```python
from build123d import *

# Parameters (mm, degrees)
SKETCH1_W           = 15.25
SKETCH1_H           = 10
SKETCH1_R           = 1.15
SKETCH1_R_2         = 0.381
BOSS_EXTRUDE1_DEPTH = 1.5
FILLET2_R           = 2


with BuildPart() as part:
    # Sketch1 → Boss-Extrude1 (new body)
    with BuildSketch(Plane(origin=(0, 0, 0), x_dir=(1, 0, 0), z_dir=(0, 1, 0))):
        with Locations((7.625, 5)):
            Rectangle(SKETCH1_W, SKETCH1_H)
        with Locations(Location((12.755741127, 5, 0), (0, 0, 270))):
            Circle(SKETCH1_R, mode=Mode.SUBTRACT)
        with Locations(Location((2, 6.27, 0), (0, 0, 270))):
            Circle(SKETCH1_R_2, mode=Mode.SUBTRACT)
        with Locations(Location((2, 3.73, 0), (0, 0, 270))):
            Circle(SKETCH1_R_2, mode=Mode.SUBTRACT)
        with Locations(Location((2, 1.19, 0), (0, 0, 270))):
            Circle(SKETCH1_R_2, mode=Mode.SUBTRACT)
        with Locations(Location((2, 8.81, 0), (0, 0, 270))):
            Circle(SKETCH1_R_2, mode=Mode.SUBTRACT)
    extrude(amount=BOSS_EXTRUDE1_DEPTH)

    # Fillet2
    fillet2_edges = [part.edges().sort_by_distance(p)[0] for p in [
        (15.25, 0.75, -10),
        (15.25, 0.75, 0),
    ]]
    fillet(fillet2_edges, radius=FILLET2_R)


solid = part.part
```
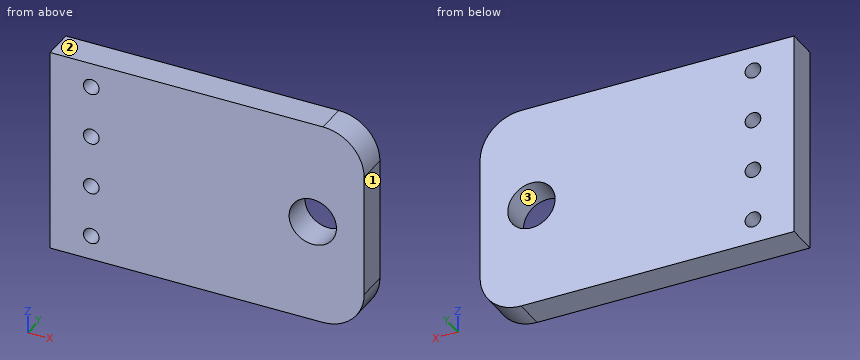
The listing builds one solid part. Answer for the finished solid, in the listing's coordinates (mm). Face numbers are marked on the shaded views. Round coordinates to 2 decimals unless told otherwise and drop trailing zeros. Order: outer loops, then holes, each group sorted by start corner. A loop starts at its lowest first (then second) coordinate and runs counter-clockwise, first axis right, second up. Notation, with made-up numbers: (28, 9) - (65, 9) arc R25 cw to (65, 34) - close; hole circle Ø11 at (80, -7). An arc over 180 degrees is marked (long way). Put each result on its own line as item: value. Start each with the question number.
(1) Determine the mould class of the marked faces 1, 2 and 3 for opening direction X: released by +X, released by -X, zero draft, split by the parting line, or undercut.
(2) Straight lines are drawn through the part: probe 1 along X at (y, z) = (1.45, -6.25); probe 2 along X at (y, z) = (0.3, -4); probe 3 along X at (y, z) = (0.95, -8.81). For each, find the intervals that lie inside material, in ascending order. Write a range as from..to.
(3) Find section B-B (z = -8.81). Give the vertices of the cut face in (x, y), plus the area to 3 significant figures.
(4) Find section A-A (x = 2). Give the vertices of the cut face in (y, z).
(5) Find section C-C (y = 0.9). Give the vertices of the cut face in (x, z), plus the area to 3 significant figures.
(6) Find section D-D (x = 14.25). Give the vertices of the cut face in (y, z), plus the area to 3 significant figures.
Reply:
1. face 1: released by +X
1. face 2: zero draft
1. face 3: undercut
2. probe 1: 0..1.62, 2.38..15.25
2. probe 2: 0..1.73, 2.27..12.19, 13.32..15.25
2. probe 3: 0..1.62, 2.38..15.08
3. outline: (0, 0) - (1.62, 0) - (1.62, 1.5) - (0, 1.5) - close; (2.38, 0) - (15.08, 0) - (15.08, 1.5) - (2.38, 1.5) - close
3. area: 21.5 mm^2
4. outline: (0, -10) - (1.5, -10) - (1.5, -9.19) - (0, -9.19) - close; (0, -8.43) - (1.5, -8.43) - (1.5, -6.65) - (0, -6.65) - close; (0, -5.89) - (1.5, -5.89) - (1.5, -4.11) - (0, -4.11) - close; (0, -3.35) - (1.5, -3.35) - (1.5, -1.57) - (0, -1.57) - close; (0, -0.81) - (1.5, -0.81) - (1.5, 0) - (0, 0) - close
5. outline: (0, -10) - (13.25, -10) arc R2 ccw to (15.25, -8) - (15.25, -2) arc R2 ccw to (13.25, 0) - (0, 0) - close; hole circle Ø0.76 at (2, -8.81); hole circle Ø0.76 at (2, -6.27); hole circle Ø0.76 at (2, -3.73); hole circle Ø0.76 at (2, -1.19); hole circle Ø2.3 at (12.76, -5)
5. area: 145 mm^2
6. outline: (0, -9.73) - (1.5, -9.73) - (1.5, -0.27) - (0, -0.27) - close
6. area: 14.2 mm^2
